from build123d import *

# Parameters (mm, degrees)
F1_DEPTH = 25.4


with BuildPart() as f1:
    # F0 (on Front) → F1 (new body)
    with BuildSketch(Plane.XZ):
        with BuildLine():
            Line((-36.4322289824, 12.1776238084), (-26.3680759817, 19.6250956506))
            Line((-26.3680759817, 19.6250956506), (-30.7963024825, 6.9442642853))
            Line((-30.7963024825, 6.9442642853), (-14.6936606616, -26.8712826073))
            Line((-14.6936606616, -26.8712826073), (1.6102636, 6.9442642853))
            Line((1.6102636, 6.9442642853), (-3.0192458071, 19.4238107651))
            Line((-3.0192458071, 19.4238107651), (8.0513199791, 11.5737747401))
            add(Edge.make_bspline(
                [(-8.539903909, -72.529733181), (-5.5298175025, -67.4291319873), (0.671369104, -56.9212011388), (7.5010896056, -38.6584394427), (8.8485062582, -6.0565384462), (8.2888064124, 6.3216018094), (8.0513199791, 11.5737747401)],
                knots=[0, 0, 0, 0, 0.2265678753, 0.466760579, 0.7737409987, 1, 1, 1, 1], degree=3))
            add(Edge.make_bspline(
                [(13.2846795022, -36.7341525853), (12.7159700105, -41.9814211739), (11.4137758116, -53.9962772925), (-1.3503029933, -65.8518595611), (-8.539903909, -72.529733181)],
                knots=[0, 0, 0, 0, 0.4367317042, 1, 1, 1, 1], degree=3))
            Line((13.2846795022, -36.7341525853), (13.2846795022, 13.1840375252))
            Line((13.2846795022, 13.1840375252), (0, 23.2481881976))
            Line((0, 23.2481881976), (3.0102304372, 23.5418692159))
            Line((3.0102304372, 23.5418692159), (35.4457411612, -3.2115069692))
            add(Edge.make_bspline(
                [(22.9310896248, -53.2794632018), (25.4561163969, -49.6894712594), (31.2619106567, -41.435002498), (36.0497072594, -17.3833263421), (35.6284960933, -7.4997772809), (35.4457411612, -3.2115069692)],
                knots=[0, 0, 0, 0, 0.3034813899, 0.6977947842, 1, 1, 1, 1], degree=3))
            add(Edge.make_bspline(
                [(42.8732857108, 3.7237356883), (42.9419768966, -0.6242385053), (43.089385872, -9.9548449559), (41.8552231799, -27.387745044), (35.8065129434, -45.2180128452), (27.0667549953, -50.6900756336), (22.9310896248, -53.2794632018)],
                knots=[0, 0, 0, 0, 0.2301910986, 0.4939823591, 0.7605517628, 1, 1, 1, 1], degree=3))
            Line((42.8732857108, 3.7237356883), (35.0232459605, 3.7237356883))
            Line((35.0232459605, 3.7237356883), (7.4474713765, 26.4687165618))
            Line((7.4474713765, 26.4687165618), (1.4089808101, 28.6828298122))
            Line((1.4089808101, 28.6828298122), (5.4076748606, 29.6522101201))
            Line((5.4076748606, 29.6522101201), (24.194162339, 18.4860005975))
            Line((24.194162339, 18.4860005975), (43.106447074, 23.0707965754))
            add(Edge.make_bspline(
                [(26.2252576649, 74.9779269099), (29.6698417944, 71.8623759308), (37.3610362325, 64.9058588415), (46.4578230677, 43.2829715579), (44.2058474785, 29.7012890641), (43.106447074, 23.0707965754)],
                knots=[0, 0, 0, 0, 0.293358708, 0.6550221388, 1, 1, 1, 1], degree=3))
            add(Edge.make_bspline(
                [(26.2252576649, 74.9779269099), (28.3474149897, 71.5501339246), (33.0834738819, 63.9002630792), (39.3930720831, 44.8851357539), (38.203019559, 34.160136648), (37.6399233937, 29.0853977203)],
                knots=[0, 0, 0, 0, 0.2995825373, 0.6685840504, 1, 1, 1, 1], degree=3))
            Line((37.6399233937, 29.0853977203), (22.2586813173, 26.1241192863))
            Line((22.2586813173, 26.1241192863), (6.6423402168, 36.9354337454))
            Line((6.6423402168, 36.9354337454), (0, 35.3251695633))
            Line((0, 35.3251695633), (3.6230948754, 40.5585281551))
            Line((3.6230948754, 40.5585281551), (19.9270192534, 38.7469828129))
            Line((19.9270192534, 38.7469828129), (28.1796231866, 63.5047927499))
            Line((28.1796231866, 63.5047927499), (9.2590199783, 73.1663778424))
            Line((9.2590199783, 73.1663778424), (22.5436985493, 61.6932436824))
            Line((22.5436985493, 61.6932436824), (17.7129078656, 44.1816225648))
            Line((17.7129078656, 44.1816225648), (1.8115479033, 45.993167907))
            Line((1.8115479033, 45.993167907), (-6.0384911485, 38.5456979275))
            Line((-6.0384911485, 38.5456979275), (-4.204464145, 43.6895005405))
            Line((-4.204464145, 43.6895005405), (-12.1035818011, 48.2374802232))
            add(Edge.make_bspline(
                [(-12.1035818011, 48.2374802232), (-11.2764509271, 46.8880557358), (-9.6011168855, 44.1548283208), (-9.2676791017, 40.8445549043), (-9.0988632253, 39.1685999437)],
                knots=[0, 0, 0, 0, 0.4937110172, 1, 1, 1, 1], degree=3))
            Line((-9.0988632253, 39.1685999437), (-12.1035818011, 42.2694329172))
            Line((-12.1035818011, 42.2694329172), (-14.4923776388, 39.9546809494))
            Line((-14.4923776388, 39.9546809494), (-17.712906003, 41.9675111771))
            Line((-17.712906003, 41.9675111771), (-20.3295852989, 40.1559621096))
            add(Edge.make_bspline(
                [(-17.8483948112, 48.476845026), (-18.4749692932, 46.9327465619), (-19.6605585437, 44.0110403751), (-20.115212391, 41.3912256195), (-20.3295852989, 40.1559621096)],
                knots=[0, 0, 0, 0, 0.5284920404, 1, 1, 1, 1], degree=3))
            Line((-17.8483948112, 48.476845026), (-25.4624815705, 43.7478435523))
            Line((-25.4624815705, 43.7478435523), (-23.7513966858, 38.3444167674))
            Line((-23.7513966858, 38.3444167674), (-31.6014327109, 45.993167907))
            Line((-31.6014327109, 45.993167907), (-47.3015084863, 43.9803414047))
            Line((-47.3015084863, 43.9803414047), (-51.729734987, 61.8945285678))
            Line((-51.729734987, 61.8945285678), (-39.2501913011, 73.3676627278))
            Line((-39.2501913011, 73.3676627278), (-57.5669445097, 63.1022304296))
            Line((-57.5669445097, 63.1022304296), (-49.9181896448, 38.948263973))
            Line((-49.9181896448, 38.948263973), (-33.4129817784, 40.5585281551))
            Line((-33.4129817784, 40.5585281551), (-29.3873213232, 35.5264544487))
            Line((-29.3873213232, 35.5264544487), (-36.8347913027, 37.1367186308))
            Line((-36.8347913027, 37.1367186308), (-52.3335859179, 26.267433539))
            Line((-52.3335859179, 26.267433539), (-67.2285333276, 29.2866788805))
            add(Edge.make_bspline(
                [(-56.2034733593, 73.6641660333), (-61.1444043649, 64.9834714788), (-70.1639673597, 49.1370507769), (-68.1425947811, 35.4678635333), (-67.2285333276, 29.2866788805)],
                knots=[0, 0, 0, 0, 0.5478015962, 1, 1, 1, 1], degree=3))
            add(Edge.make_bspline(
                [(-56.2034733593, 73.6641660333), (-59.3451927185, 71.1733267977), (-66.60773384, 65.4153897232), (-75.5386939948, 43.9944008325), (-73.6153653527, 29.9834038748), (-72.6631730795, 23.0469070375)],
                knots=[0, 0, 0, 0, 0.2779550238, 0.6425334536, 1, 1, 1, 1], degree=3))
            Line((-72.6631730795, 23.0469070375), (-53.9438501, 18.2161126286))
            Line((-53.9438501, 18.2161126286), (-34.8219648004, 31.0982260853))
            Line((-34.8219648004, 31.0982260853), (-30.9975855052, 29.2866788805))
            Line((-30.9975855052, 29.2866788805), (-37.8412082791, 26.6700014472))
            Line((-37.8412082791, 26.6700014472), (-65.4169842601, 2.7173208073))
            Line((-65.4169842601, 2.7173208073), (-71.8580409884, 2.7173208073))
            add(Edge.make_bspline(
                [(-71.8580409884, 2.7173208073), (-71.8323808051, -0.6743290469), (-71.7707586489, -8.819273873), (-72.3514628162, -31.1556090613), (-63.3168519567, -46.9122797723), (-56.4054375512, -51.3169694206), (-53.3260814846, -53.2794632018)],
                knots=[0, 0, 0, 0, 0.2151105122, 0.5165814068, 0.784614568, 1, 1, 1, 1], degree=3))
            add(Edge.make_bspline(
                [(-53.3260814846, -53.2794632018), (-56.0259363166, -49.0184463117), (-61.9673181702, -39.6415242162), (-65.9171343123, -16.4717993255), (-65.7087984168, -6.8839300031), (-65.6182616949, -2.7173208073)],
                knots=[0, 0, 0, 0, 0.3201642849, 0.7045631676, 1, 1, 1, 1], degree=3))
            Line((-65.6182616949, -2.7173208073), (-34.4193968922, 23.2481881976))
            Line((-34.4193968922, 23.2481881976), (-30.393736437, 23.2481881976))
            Line((-30.393736437, 23.2481881976), (-43.0745668709, 12.3789058998))
            Line((-43.0745668709, 12.3789058998), (-43.0745668709, -39.5521149039))
            add(Edge.make_bspline(
                [(-43.0745668709, -39.5521149039), (-41.8262985236, -43.8907788266), (-39.2078569373, -52.9918171315), (-29.1900934235, -67.2654171685), (-22.8102743449, -70.9265355416), (-20.0165621936, -72.529733181)],
                knots=[0, 0, 0, 0, 0.3386642474, 0.7104021751, 1, 1, 1, 1], degree=3))
            add(Edge.make_bspline(
                [(-20.0165621936, -72.529733181), (-23.3797839012, -67.1871365793), (-30.2770206692, -56.2306320954), (-36.3841217142, -37.273284048), (-39.4008360571, -2.9353787105), (-37.2794445977, 7.8644993682), (-36.4322289824, 12.1776238084)],
                knots=[0, 0, 0, 0, 0.2324437246, 0.4766915604, 0.7910074166, 1, 1, 1, 1], degree=3))
        make_face()
    extrude(amount=F1_DEPTH)


solid = f1.part
For this review, take the finished solid that the model builds, in its own axes (mm). A direction names the side the tool comes from. Coordinates: 2 decimals unless noted, no trailing zeros. Return JSON: item names as keys, results as strings.
1. We need section A-A on x = 32. State how many separate pieces and enclosed holes the cut face has, and give its area (3 significant figures).
Answer block:
{"separate pieces": "4", "enclosed holes": "0", "area": "776 mm²"}
2. The part is to be moulded in two halves that separate along X. For faces 1 (the flat face through (33.518, -12.522, 20.746)), 2 (the flat face through (-15, -25.4, 7)), 3 (the flat face through (30.057, -12.522, 27.625)), say which applies: +X half, -X half, draft (parallel to the pull), parting line (faces both ways), or undercut.
Answer block:
{"face 1": "+X half", "face 2": "draft", "face 3": "undercut"}
3. For pin 1 Ø6 at (x, y) = (-60.5, -15) entering from -Z; pin 2 Ø8 at (y, z) = (-10.5, 52) entering from +X; pin 3 Ø7.5 at (y, z) = (-18, -15) entering from +X, all flat-tipped, find the tip position at first contact; note any pin that passes through.
Answer block:
{"pin 1": "z = -50.5", "pin 2": "x = 43.42", "pin 3": "x = 42.82"}
4. Machinability: for faces 4 (the flat face through (14.669, -12.522, 24.147)), 5 (the flat face through (-15, 0, 7)), which of the approach directions +Z, -Z, +X, -X, +Y, -Y give a long, thin tool a straight path to every point of the face, cutting with its end or side? Answer none if there is none.
Answer block:
{"face 4": "+Y, -Y", "face 5": "+Z, -Z, +X, -X, +Y"}
5. For line 1 (X direction, y = -10, z = -8.5); line 2 (Z direction, x = -58.5, y = -0.75); line 3 (X direction, y = -19.75, z = -35), list the stretches that pass through material, from the lowest coordinate up. Write a range as from..to.
Answer block:
{"line 1": "-71.86..-65.69, -43.07..-38.31, -23.44..-5.84, 8.47..13.28, 35.62..42.9", "line 2": "-49.76..-44.4, 3.21..8.73, 19.39..27.52, 69.61..71.82", "line 3": "-69.14..-62.06, -43.07..-35.74, 6.69..13.28, 32..38.97"}
